```python
from build123d import *

# Parameters (mm, degrees)
F2_R    = 2
F3_SIZE = 0.8


with BuildPart() as f1:
    # F0 (on Top) → F1 (revolve)
    with BuildSketch(Plane.XY):
        Polygon((12, 8.75), (12, 0), (78, 0), (78, 8.75), (90, 8.75), (90, 24.9), (0, 24.9), (0, 8.75), align=None)
    revolve(axis=Axis((45, 0, 0), (-1, 0, 0)))

    # F2
    f2_edges = [f1.edges().sort_by_distance(p)[0] for p in [
        (0, -24.9, 0),
        (90, -24.9, 0),
    ]]
    fillet(f2_edges, radius=F2_R)

    # F3
    f3_edges = [f1.edges().sort_by_distance(p)[0] for p in [
        (0, -8.75, 0),
        (90, -8.75, 0),
    ]]
    chamfer(f3_edges, length=F3_SIZE)


solid = f1.part
```
Can you work these out from the model? Positions are in its coordinate system, mm. A direction names the side the tool comes from. Coordinates: 2 decimals unless noted, no trailing zeros. Write each loop counter-clockwise with the first axis right and the second up, starting at its lowest first coordinate (ties: lowest second). Pieces come first, ordered by that corner, then holes. Notation, with made-up numbers: (61.5, -23) - (111.5, -23) arc R8 cw to (111.5, -14) - close; hole circle Ø1 at (19.25, 74). An arc over 180 degrees is marked (long way). Return JSON: item names as keys, results as strings.
Q1. I'm going to push flat-ended pins straight in: pin 1 Ø6 at (x, y) = (10, 8) entering from -Z; pin 2 Ø2 at (x, z) = (38, 19.5) entering from +Y; pin 3 Ø12 at (x, y) = (68, -16) entering from +Z. Where does each tip first touch, or does it pass through?
Computed values:
{"pin 1": "stops at z = -24.39", "pin 2": "stops at y = 16.67", "pin 3": "stops at z = 22.8"}
Q2. On a 3-axis mill with a long thin cutter (end or side, diameter ignored), from which of +Z, -Z, +X, -X, +Y, -Y can I reach the whole of each face in a straight line? I mean faces 5 (the flat face through (90, -10, 0)), 6 (the flat face through (78, 0, 0)), 7 (the cylindrical face through (6.478, -6.944, 5.324)). Say none if no direction works.
Computed values:
{"face 5": "+Z, -Z, +X, +Y, -Y", "face 6": "+X", "face 7": "-X"}
Q3. If we section it at C-C (x = 66.5): Please give me the cut outline in (y, z), then the cut area to 3 significant figures.
Computed values:
{"outline": "circle Ø49.8 at (0, 0)", "area": "1,950 mm2"}
Q4. Thinking about a two-plate mould opening in Y: for faces 1 (the flat face through (12, 0, 0)), 2 (the cylindrical face through (83.678, -6.944, 5.324)), 3 (the cylindrical face through (44.4, -18.35, -16.83)), 4 (the flat face through (0, 10, 0)), which applies, +Y half, -Y half, draft (parallel to the pull), parting line (faces both ways), or undercut?
Computed values:
{"face 1": "undercut", "face 2": "undercut", "face 3": "parting line", "face 4": "draft"}
Q5. If we section it at A-A (z = 0): Please give me the cut outline in (x, y), then the cut area to 3 significant figures.
Computed values:
{"outline": "(0, -22.9) arc R2 ccw to (2, -24.9) - (88, -24.9) arc R2 ccw to (90, -22.9) - (90, -9.55) - (89.2, -8.75) - (78, -8.75) - (78, 8.75) - (89.2, 8.75) - (90, 9.55) - (90, 22.9) arc R2 ccw to (88, 24.9) - (2, 24.9) arc R2 ccw to (0, 22.9) - (0, 9.55) - (0.8, 8.75) - (12, 8.75) - (12, -8.75) - (0.8, -8.75) - (0, -9.55) - close", "area": "4,060 mm2"}
Q6. Please list where these lines run through material, in increasing order: L1, parallel to Y at x = 81.75, z = 0; L2, parallel to Z at x = 9, y = 5. Write a range as from..to.
Computed values:
{"L1": "y = -24.9..-8.75, 8.75..24.9", "L2": "z = -24.39..-7.18, 7.18..24.39"}
